The listing builds one solid part. Answer for the finished solid, in the listing's coordinates (mm). A direction names the side the tool comes from. Give positions to 0.01 mm unless a question says otherwise; leave off trailing zeros. Loops run counter-clockwise (first coordinate to the right, second up) from the corner with the lowest first, then second, coordinate; pieces in that order, holes last. Notation, with made-up numbers: (-13.5, 12.25) - (15.5, 12.25) arc R16 ccw to (15.5, 31.25) - close; hole circle Ø3 at (-28, 31). An arc over 180 degrees is marked (long way). One line per item, written item: value. Start each with the question number.
from build123d import *

# Parameters (mm, degrees)
SKETCH1_R           = 8
BOSS_EXTRUDE1_DEPTH = 3.3
SKETCH2_R           = 5.5
BOSS_EXTRUDE2_DEPTH = 9
SKETCH3_R           = 3
CUT_EXTRUDE3_DEPTH  = 4.3
CUT_EXTRUDE3_TAPER  = -45
SKETCH4_R           = 3
CUT_EXTRUDE4_DEPTH  = 13.3000001


with BuildPart() as part:
    # Sketch1 → Boss-Extrude1 (new body)
    with BuildSketch(Plane.XY):
        Circle(SKETCH1_R)
    extrude(amount=BOSS_EXTRUDE1_DEPTH)

    # Sketch2 → Boss-Extrude2 (add)
    with BuildSketch(Plane.XY.offset(3.3)):
        Circle(SKETCH2_R)
    extrude(amount=BOSS_EXTRUDE2_DEPTH)

    # Sketch3 → Cut-Extrude3 (cut, through all)
    with BuildSketch(Plane.XY.offset(3.3)):
        Circle(SKETCH3_R)
    extrude(amount=-CUT_EXTRUDE3_DEPTH, taper=CUT_EXTRUDE3_TAPER, mode=Mode.SUBTRACT)

    # Sketch4 → Cut-Extrude4 (cut, through all)
    with BuildSketch(Plane.XY.offset(12.3)):
        Circle(SKETCH4_R)
    extrude(amount=-CUT_EXTRUDE4_DEPTH, mode=Mode.SUBTRACT)


solid = part.part
1. A cutting plane is placed at A-A (x = 0). Determine the outline of the cut face in (y, z), plus the area to 3 significant figures.
2. Determine the mould class of faces 3 (the cylindrical face through (-3, 0, 8)), 4 (the conical face through (-0.7, -3.13, 3.09)), 5 (the cylindrical face through (-1.19, -5.37, 7.74)), 6 (the flat face through (2.4, -2.4, 12.3)) for opening direction Y: released by +Y, released by -Y, zero draft, split by the parting line, or undercut.
3. A cutting plane is placed at B-B (z = 11.25). Determine the outline of the cut face in (x, y), plus the area to 3 significant figures.
4. Flat-ended cylindrical pins translate along their axes: pin 1 (2 mm diameter, centred on y = 5, z = 1.5, fed in from -X); pin 2 (4 mm diameter, centred on y = 2.5, z = 3.5, fed in from -X); pin 3 (8 mm diameter, centred on x = 1.5, y = -0.5, fed in from -Z); pin 4 (3 mm diameter, centred on x = -6.5, y = 4.5, fed in from -Z). Find the tip coordinate at first contact, or state that the pin passes through.
5. For faces 1 (the flat face through (1.7, 5.4, 3.3)), 2 (the flat face through (0, -6.5, 0)), determine the directions among +Z, -Z, +X, -X, +Y, -Y from which every point of the face is accessible in a straight line to the end or side of a thin tool.
6. Find the intervals of material crossed by L1, parallel to Y at x = 0, z = 7.25; L2, parallel to Z at x = -0.5, y = -7.25; L3, parallel to X at y = -2, z = 7.5, in increasing order. Write a range as [from, to].
Results below:
1. outline: (-8, 0) - (-6.3, 0) - (-3, 3.3) - (-3, 12.3) - (-5.5, 12.3) - (-5.5, 3.3) - (-8, 3.3) - close; (3, 3.3) - (6.3, 0) - (8, 0) - (8, 3.3) - (5.5, 3.3) - (5.5, 12.3) - (3, 12.3) - close
1. area: 67.1 mm^2
2. face 3: undercut
2. face 4: undercut
2. face 5: split by the parting line
2. face 6: zero draft
3. outline: circle Ø11 at (0, 0); hole circle Ø6 at (0, 0)
3. area: 66.8 mm^2
4. pin 1: stops at x = -6.93
4. pin 2: stops at x = -7.98
4. pin 3: stops at z = 0.72
4. pin 4: stops at z = 0
5. face 1: +Z
5. face 2: -Z, +X, -X, +Y, -Y
6. L1: y = [-5.5, -3], [3, 5.5]
6. L2: z = [0, 3.3]
6. L3: x = [-5.12, -2.24], [2.24, 5.12]
